Design review of the part built by this model. Coordinates are the model's own, in mm. Face numbers are marked on the shaded views. A direction names the side the tool comes from. Give positions to 0.01 mm unless a question says otherwise; leave off trailing zeros. Order: outer loops, then holes, each group sorted by start corner. A loop starts at its lowest first (then second) coordinate and runs counter-clockwise, first axis right, second up. Notation, with made-up numbers: (-35.5, 17.5) -> (5.5, 17.5) arc R8 ccw to (5.5, 23.5) -> close; hole circle Ø7 at (-26, 88). An arc over 180 degrees is marked (long way). One line per item, written item: value. Start each with the question number.
1) The part is to be moulded in two halves that separate along Y. For the marked faces 3, 4 and 5, say which applies: released by +Y, released by -Y, zero draft, split by the parting line, or undercut.
2) Consider section A-A (z = 38). State the section outline as (x, y) points.
3) Consider section D-D (x = 6). State the section outline as (y, z) points, plus the area to 3 significant figures.
4) Consider section C-C (y = 8.5). State the section outline as (x, z) points.
5) Consider section B-B (x = 35). State the section outline as (y, z) points, plus the area to 3 significant figures.
6) Tool access review of the marked faces 1 and 2: name each direction out of +Z, -Z, +X, -X, +Y, -Y from which nothing blocks a thin tool from reaching the whole face with its end or side.
7) Wall thickness on line 1 along X through (y, z) = (0.8, 22); line 2 along X through (y, z) = (1.25, 52); line 3 along X through (y, z) = (2.25, 25): over which ranges is each line inside the solid? List them lowest first. Write a range as from..to.
8) For pin 1 (6 mm diameter, centred on y = 17, z = 36.5, fed in from +X); pin 2 (4.5 mm diameter, centred on x = 45.5, y = 1.5, fed in from -Z); pin 3 (1.2 mm diameter, centred on x = -7.5, y = 2, fed in from +Z), all flat-tipped, find the tip position at first contact; note any pin that passes through.
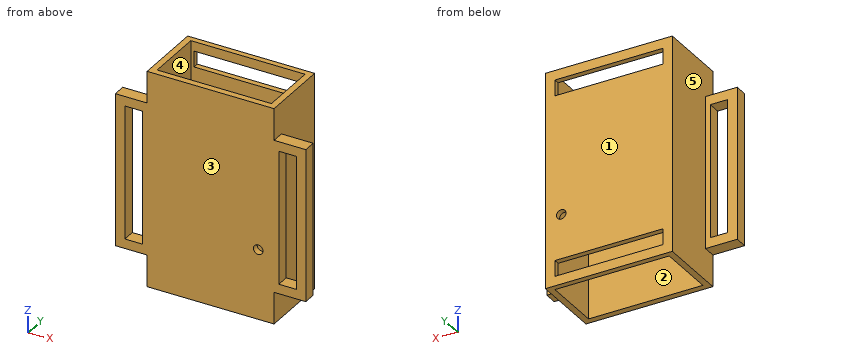
from build123d import *

# Parameters (mm, degrees)
SKETCH1_W           = 40
SKETCH1_H           = 68
SKETCH1_R           = 1.5
BOSS_EXTRUDE1_DEPTH = 22
SKETCH2_W           = 36
SKETCH2_H           = 18.265871498
CUT_EXTRUDE1_DEPTH  = 69
SKETCH3_W           = 34
SKETCH3_H           = 5
CUT_EXTRUDE2_DEPTH  = 2
SKETCH6_W           = 48
SKETCH6_H           = 4
BOSS_EXTRUDE3_DEPTH = 10
SKETCH7_W           = 5.490890851
SKETCH7_H           = 42
CUT_EXTRUDE4_DEPTH  = 10


with BuildPart() as part:
    # Sketch1 → Boss-Extrude1 (new body)
    with BuildSketch(Plane(origin=(0, 0, 0), x_dir=(1, 0, 0), z_dir=(0, 1, 0))):
        with Locations((20, -34)):
            Rectangle(SKETCH1_W, SKETCH1_H)
        with Locations((35, -22)):
            Circle(SKETCH1_R, mode=Mode.SUBTRACT)
    extrude(amount=BOSS_EXTRUDE1_DEPTH)

    # Sketch2 → Cut-Extrude1 (cut, through all)
    with BuildSketch(Plane.XY.offset(68)):
        with Locations((20, 11.132935749)):
            Rectangle(SKETCH2_W, SKETCH2_H)
    extrude(amount=-CUT_EXTRUDE1_DEPTH, mode=Mode.SUBTRACT)

    # Sketch3 → Cut-Extrude2 (cut)
    with BuildSketch(Plane(origin=(0, 22, 0), x_dir=(1, 0, 0), z_dir=(0, 1, 0))):
        with Locations((20, -62.5)):
            Rectangle(SKETCH3_W, SKETCH3_H)
        with Locations((20, -5.5)):
            Rectangle(SKETCH3_W, SKETCH3_H)
    extrude(amount=-CUT_EXTRUDE2_DEPTH, mode=Mode.SUBTRACT)

    # Sketch6 → Boss-Extrude3 (add)
    with BuildSketch(Plane(origin=(40, 0, 0), x_dir=(0, 0, -1), z_dir=(1, 0, 0))):
        with Locations((-34, 2)):
            Rectangle(SKETCH6_W, SKETCH6_H)
    boss_extrude3 = extrude(amount=BOSS_EXTRUDE3_DEPTH)

    # Sketch7 → Cut-Extrude4 (cut)
    with BuildSketch(Plane(origin=(0, 4, 0), x_dir=(1, 0, 0), z_dir=(0, 1, 0))):
        with Locations((44.254554575, -34)):
            Rectangle(SKETCH7_W, SKETCH7_H)
    cut_extrude4 = extrude(amount=-CUT_EXTRUDE4_DEPTH, mode=Mode.SUBTRACT)

    # Mirror1: Boss-Extrude3 across plane
    add(boss_extrude3.mirror(Plane(origin=(20, 0, 0), x_dir=(0, 0, 1), z_dir=(1, 0, 0))))

    # Mirror2: Cut-Extrude4 across plane
    add(cut_extrude4.mirror(Plane(origin=(20, 0, 0), x_dir=(0, 0, 1), z_dir=(1, 0, 0))), mode=Mode.SUBTRACT)


solid = part.part
Checked values:
1. face 3: released by -Y
1. face 4: undercut
1. face 5: zero draft
2. outline: (-10, 0) -> (-7, 0) -> (-7, 4) -> (-10, 4) -> close; (-1.51, 0) -> (41.51, 0) -> (41.51, 4) -> (40, 4) -> (40, 22) -> (0, 22) -> (0, 4) -> (-1.51, 4) -> close; (47, 0) -> (50, 0) -> (50, 4) -> (47, 4) -> close; hole (2, 2) -> (38, 2) -> (38, 20.27) -> (2, 20.27) -> close
3. outline: (0, 0) -> (2, 0) -> (2, 68) -> (0, 68) -> close; (20.27, 0) -> (22, 0) -> (22, 3) -> (20.27, 3) -> close; (20.27, 8) -> (22, 8) -> (22, 60) -> (20.27, 60) -> close; (20.27, 65) -> (22, 65) -> (22, 68) -> (20.27, 68) -> close
3. area: 237 mm^2
4. outline: (0, 0) -> (2, 0) -> (2, 68) -> (0, 68) -> close; (38, 0) -> (40, 0) -> (40, 68) -> (38, 68) -> close
5. outline: (0, 0) -> (2, 0) -> (2, 20.5) -> (0, 20.5) -> close; (0, 23.5) -> (2, 23.5) -> (2, 68) -> (0, 68) -> close; (20.27, 0) -> (22, 0) -> (22, 3) -> (20.27, 3) -> close; (20.27, 8) -> (22, 8) -> (22, 20.5) -> (20.27, 20.5) -> close; (20.27, 23.5) -> (22, 23.5) -> (22, 60) -> (20.27, 60) -> close; (20.27, 65) -> (22, 65) -> (22, 68) -> (20.27, 68) -> close
5. area: 225 mm^2
6. face 1: +Z, -Z, +X, -X, +Y
6. face 2: +Z, -Z
7. line 1: x = -10..-7, -1.51..33.5, 36.5..41.51, 47..50
7. line 2: x = -10..-7, -1.51..41.51, 47..50
7. line 3: x = -10..-7, -1.51..2, 38..41.51, 47..50
8. pin 1: stops at x = 40
8. pin 2: stops at z = 10
8. pin 3: stops at z = 58
